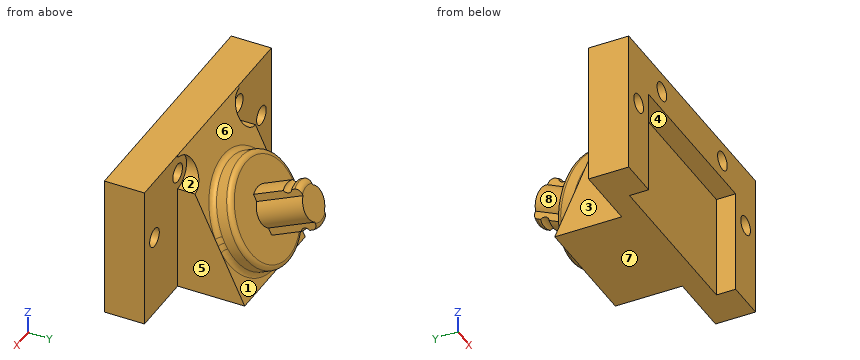
from build123d import *

# Parameters (mm, degrees)
BOSS_EXTRUDE1_DEPTH = 7.5
SKETCH8_W           = 35.6
SKETCH8_H           = 5.75
BOSS_EXTRUDE4_DEPTH = 5.6
BOSS_EXTRUDE5_DEPTH = 8.5
SKETCH3_R           = 7.86
BOSS_EXTRUDE2_DEPTH = 3
FILLET4_R           = 0.7
BOSS_EXTRUDE3_DEPTH = 7.32
SKETCH6_R           = 0.715
CUT_EXTRUDE2_DEPTH  = 20.15
FILLET5_R           = 0.8
SKETCH9_R           = 1.35
CUT_EXTRUDE3_DEPTH  = 6.75
SKETCH12_R          = 2.5
CUT_EXTRUDE4_DEPTH  = 17.312326385


with BuildPart() as part:
    # Sketch1 → Boss-Extrude1 (new body, symmetric)
    with BuildSketch(Plane.XY):
        Polygon((-17.8, 5.75), (17.8, 5.75), (17.8, 0), (12.2, 0), (12.2, 2.75), (-12.2, 2.75), (-12.2, 0), (-17.8, 0), align=None)
    extrude(amount=BOSS_EXTRUDE1_DEPTH, both=True)

    # Sketch8 → Boss-Extrude4 (add)
    with BuildSketch(Plane.XY.offset(7.5)):
        with Locations((0, 2.875)):
            Rectangle(SKETCH8_W, SKETCH8_H)
    extrude(amount=BOSS_EXTRUDE4_DEPTH)

    # Sketch11 → Boss-Extrude5 (add, symmetric)
    with BuildSketch(Plane(origin=(0, 0, 0), x_dir=(0, 0, -1), z_dir=(1, 0, 0))):
        Polygon((-13.1, 5.75), (7.5, 15.355937758), (7.5, 5.75), align=None)
    extrude(amount=BOSS_EXTRUDE5_DEPTH, both=True)

    # Sketch3 → Boss-Extrude2 (add)
    with BuildSketch(Plane(origin=(0, -0.825909529, 27.202083493), x_dir=(1, 0, 0), z_dir=(0, -0.906307787, -0.422618262))):
        with Locations((0, -29.289512668)):
            Circle(SKETCH3_R)
    extrude(amount=-BOSS_EXTRUDE2_DEPTH)

    # Fillet4
    fillet4_edges = [part.edges().sort_by_distance(p)[0] for p in [
        (-7.86, 14.271296763, 1.924624869),
        (-7.86, 11.552373402, 0.656770083),
    ]]
    fillet(fillet4_edges, radius=FILLET4_R)

    # Sketch5 → Boss-Extrude3 (add)
    with BuildSketch(Plane(origin=(0, 12.459528841, 5.809973716), x_dir=(1, 0, 0), z_dir=(0, 0.906307787, 0.422618262))):
        with BuildLine():
            Line((1.35, 6.277366133), (1.35, 7.363873413))
            ThreePointArc((1.35, 7.363873413), (0, 7.647008125), (-1.35, 7.363873413))
            Line((-1.35, 7.363873413), (-1.35, 6.277366133))
            ThreePointArc((-1.35, 6.277366133), (-2.405, 4.287008125), (-1.35, 2.296650117))
            Line((-1.35, 2.296650117), (-1.35, 1.210142838))
            ThreePointArc((-1.35, 1.210142838), (0, 0.927008125), (1.35, 1.210142838))
            Line((1.35, 1.210142838), (1.35, 2.296650117))
            ThreePointArc((1.35, 2.296650117), (2.405, 4.287008125), (1.35, 6.277366133))
        make_face()
    extrude(amount=BOSS_EXTRUDE3_DEPTH)

    # Sketch6 → Cut-Extrude2 (cut, through all)
    with BuildSketch(Plane(origin=(1.35, 0, 0), x_dir=(0, 0, -1), z_dir=(1, 0, 0))):
        with Locations((-7.239279099, 17.71817222)):
            Circle(SKETCH6_R)
        with Locations((-1.14889077, 20.558166939)):
            Circle(SKETCH6_R)
    extrude(amount=-CUT_EXTRUDE2_DEPTH, mode=Mode.SUBTRACT)

    # Fillet5
    fillet5_edges = [part.edges().sort_by_distance(p)[0] for p in [
        (0, 19.485472405, 8.063384709),
        (0, 22.325467124, 1.97299638),
    ]]
    fillet(fillet5_edges, radius=FILLET5_R)

    # Sketch9 → Cut-Extrude3 (cut, through all)
    with BuildSketch(Plane(origin=(0, 5.75, 0), x_dir=(1, 0, 0), z_dir=(0, 1, 0))):
        with Locations((-8.5, -10.3)):
            Circle(SKETCH9_R)
        with Locations((-15, -4.3)):
            Circle(SKETCH9_R)
        with Locations((8.5, -10.3)):
            Circle(SKETCH9_R)
        with Locations((15, -4.3)):
            Circle(SKETCH9_R)
    extrude(amount=-CUT_EXTRUDE3_DEPTH, mode=Mode.SUBTRACT)

    # Sketch12 → Cut-Extrude4 (cut, through all)
    with BuildSketch(Plane(origin=(0, 5.75, 0), x_dir=(-1, 0, 0), z_dir=(0, 1, 0))):
        with Locations((8.5, 10.3)):
            Circle(SKETCH12_R)
        with Locations((-8.5, 10.3)):
            Circle(SKETCH12_R)
    extrude(amount=CUT_EXTRUDE4_DEPTH, mode=Mode.SUBTRACT)


solid = part.part
The model under review builds one solid part; all positions refer to its coordinate system, in mm. Face numbers are marked on the shaded views. A direction names the side the tool comes from. Give positions to 0.01 mm unless a question says otherwise; leave off trailing zeros. Loops run counter-clockwise (first coordinate to the right, second up) from the corner with the lowest first, then second, coordinate; pieces in that order, holes last. Notation, with made-up numbers: (12, -30) -> (68, -30) arc R36 cw to (68, 4) -> close; hole circle Ø5 at (37.5, 36). An arc over 180 degrees is marked (long way). Answer as a JSON object with one key per item and string values. Group by question number.
Q1. Take a section at D-D (x = -13). Write out the cut boundary in (y, z), plus the area to 3 significant figures.
Q2. Take a section at A-A (x = 15). Write out the cut boundary in (y, z).
Q3. Draft analysis for pull direction Z (two halves, no side actions). For the marked faces 6, 7 and 8, state which applies: pulls with the +Z half, pulls with the -Z half, needs draft (parallel to the pull), parting line crosses it, or undercut.
Q4. Take a section at B-B (y = 2). Write out the cut boundary in (x, z), plus the area to 3 significant figures.
Q5. Take a section at C-C (z = 10.3). Write out the cut boundary in (x, y).
Q6. Insertion check: pin 1 (12 mm diameter, centred on y = 13, z = -4, fed in from +X); pin 2 (1 mm diameter, centred on x = 11.5, z = 8.5, fed in from +Y); pin 3 (4.5 mm diameter, centred on y = 17.5, z = 1.5, fed in from -X) (3 decimals). Each pin has a flat end and moves straight along its axis. Give the tip position at first contact, or say it passes through.
Q7. Tool access review of the marked faces 1, 2, 3, 4 and 5: name each direction out of +Z, -Z, +X, -X, +Y, -Y from which nothing blocks a thin tool from reaching the whole face with its end or side.
Q8. Wall thickness on line 1 along X through (y, z) = (1.35, 10.3); line 2 along X through (y, z) = (1.85, 4.3); line 3 along Z through (x, y) = (8.5, 2.5): over which ranges is each line inside the solid? List them lowest first.
Answer below:
{
 "1": {"outline": "(0, -7.5) -> (5.75, -7.5) -> (5.75, 13.1) -> (0, 13.1) -> close", "area": "118 mm2"},
 "2": {"outline": "(0, -7.5) -> (5.75, -7.5) -> (5.75, 2.95) -> (0, 2.95) -> close; (0, 5.65) -> (5.75, 5.65) -> (5.75, 13.1) -> (0, 13.1) -> close"},
 "3": {"face 6": "pulls with the +Z half", "face 7": "pulls with the -Z half", "face 8": "undercut"},
 "4": {"outline": "(-17.8, -7.5) -> (-12.2, -7.5) -> (-12.2, 7.5) -> (12.2, 7.5) -> (12.2, -7.5) -> (17.8, -7.5) -> (17.8, 13.1) -> (-17.8, 13.1) -> close; hole circle Ø2.7 at (-15, 4.3); hole circle Ø2.7 at (-8.5, 10.3); hole circle Ø2.7 at (8.5, 10.3); hole circle Ø2.7 at (15, 4.3)", "area": "344 mm2"},
 "5": {"outline": "(-17.8, 0) -> (-9.85, 0) -> (-9.85, 5.75) -> (-17.8, 5.75) -> close; (-7.15, 0) -> (7.15, 0) -> (7.15, 5.75) -> (6, 5.75) -> (6, 7.06) -> (-6, 7.06) -> (-6, 5.75) -> (-7.15, 5.75) -> close; (9.85, 0) -> (17.8, 0) -> (17.8, 5.75) -> (9.85, 5.75) -> close"},
 "6": {"pin 1": "stops at x = 8.5", "pin 2": "stops at y = 5.75", "pin 3": "stops at x = -2.405"},
 "7": {"face 1": "+Y", "face 2": "+X, +Y", "face 3": "+Z, -Z, -X, +Y", "face 4": "-Z, -Y", "face 5": "+Z, -Z, +X, +Y"},
 "8": {"line 1": "x = -17.8 to -9.85, -7.15 to 7.15, 9.85 to 17.8", "line 2": "x = -17.8 to -16.35, -13.65 to -12.2, 12.2 to 13.65, 16.35 to 17.8", "line 3": "z = 7.5 to 8.95, 11.65 to 13.1"}
}
